Model file for the job. Use its own axes, mm. A direction names the side the tool comes from. Give positions to 0.01 mm unless a question says otherwise; leave off trailing zeros. Loops run counter-clockwise (first coordinate to the right, second up) from the corner with the lowest first, then second, coordinate; pieces in that order, holes last. Notation, with made-up numbers: M -39,-22.75 L -33,-22.75 A19 cw -33,6.25 Z; hole C 9,67 d1. An arc over 180 degrees is marked long. Use CSV: the item, a comma, the result in double quotes. Start each with the question number.
(1) Slice it at C-C on z = 15.75. List the corners of the cut face in (x, y).
(2) Wall check: line 1 along Y through (x, z) = (0, 26.1); line 2 along X through (y, z) = (-9.25, 25.65); line 3 along Y through (x, z) = (-30, 0.9). Give the ranges that are in metal, low to high. Write a range as from..to.
(3) Slice it at D-D on y = 0. State how many separate pieces and enclosed holes the cut face has, and give its area (3 significant figures).
(4) Two-plate mould, pull along Z, no slides. Class faces 4 (the face through (-15, -15, 0)), 5 (the face through (16, -16, 20)), 6 (the face through (0, -5, 28)), 7 (the face through (6.25, 0.07, 26.52)): pulls with the +Z half, pulls with the -Z half, needs draft (parallel to the pull), parting line crosses it, or undercut.
(5) Tool access for faces 1 (the face through (10.042, -20.649, 22.465)), 2 (the face through (-4, 4, 25)), 3 (the face through (-7.5, -22, 11)): list every direction of +Z, -Z, +X, -X, +Y, -Y with a clear straight run to the whole face (end or side of a thin tool).
(6) Slice it at A-A on x = 30. List the corners of the cut face in (y, z), and give its area (3 significant figures).
(7) Flat gauge pins, fed straight in: P1, Ø4, axis at y = -5.5, z = 3, coming from the -X side; P2, Ø4, axis at x = 4.5, z = 4, coming from the -Y side; P3, Ø3.5, axis at x = 0, y = -9.25, coming from the -Z side; P4, Ø7, axis at x = 0, y = 0, coming from the +Z side. Where does each tip first touch, or does it go through?
```python
from build123d import *

# Parameters (mm, degrees)
SKETCH_1_R               = 25
SKETCH_1_R_2             = 21
EXTRUDE_1_DEPTH          = 25
SKETCH_2_R               = 25
EXTRUDE_2_DEPTH          = 3
SKETCH_3_R               = 4.25
SKETCH_3_R_2             = 1.5
CUT_EXTRUDE_1_DEPTH      = 3
CUT_EXTRUDE_2_DEPTH      = 3
SKETCH_6_W               = 15
SKETCH_6_H               = 5
CUT_EXTRUDE_3_DEPTH      = 63
SKETCH_8_W               = 5
SKETCH_8_H               = 15
CUT_EXTRUDE_4_DEPTH      = 63
SKETCH_9_W               = 5
SKETCH_9_H               = 15
CUT_EXTRUDE_5_DEPTH      = 63
PATTERN_CIRCULAR_2_COUNT = 4
SKETCH_10_R              = 35
SKETCH_10_R_2            = 21
EXTRUDE_3_DEPTH          = 3
SKETCH_11_R              = 2
CUT_EXTRUDE_6_DEPTH      = 3
FILLET_1_R               = 2


with BuildPart() as part:
    # 草图1 → 凸台-拉伸1 (new body)
    with BuildSketch(Plane.XY):
        Circle(SKETCH_1_R)
        Circle(SKETCH_1_R_2, mode=Mode.SUBTRACT)
    extrude(amount=EXTRUDE_1_DEPTH)

    # 草图2 → 凸台-拉伸2 (add)
    with BuildSketch(Plane.XY.offset(25)):
        Circle(SKETCH_2_R)
    extrude(amount=EXTRUDE_2_DEPTH)

    # 草图3 → 切除-拉伸1 (cut)
    with BuildSketch(Plane.XY.offset(28)):
        Circle(SKETCH_3_R)
        with Locations((0, 9.25)):
            Circle(SKETCH_3_R_2)
        with Locations((7.75, 0)):
            Circle(SKETCH_3_R_2)
        with Locations(Location((0, -9.25, 0), (0, 0, 180))):
            Circle(SKETCH_3_R_2)
        with Locations(Location((-7.75, 0, 0), (0, 0, 180))):
            Circle(SKETCH_3_R_2)
    extrude(amount=-CUT_EXTRUDE_1_DEPTH, mode=Mode.SUBTRACT)

    # 草图4 → 切除-拉伸2 (cut)
    with BuildSketch(Plane.XY.offset(28)):
        with BuildLine():
            ThreePointArc((-17.320508076, 10), (-20, 0), (-17.320508076, -10))
            ThreePointArc((-17.320508076, -10), (-13.905444566, -10.915063509), (-12.990381057, -7.5))
            ThreePointArc((-12.990381057, -7.5), (-15, 0), (-12.990381057, 7.5))
            ThreePointArc((-12.990381057, 7.5), (-13.905444566, 10.915063509), (-17.320508076, 10))
        make_face()
        with BuildLine():
            ThreePointArc((17.320508076, 10), (20, 0), (17.320508076, -10))
            ThreePointArc((17.320508076, -10), (13.905444566, -10.915063509), (12.990381057, -7.5))
            ThreePointArc((12.990381057, -7.5), (15, 0), (12.990381057, 7.5))
            ThreePointArc((12.990381057, 7.5), (13.905444566, 10.915063509), (17.320508076, 10))
        make_face()
    extrude(amount=-CUT_EXTRUDE_2_DEPTH, mode=Mode.SUBTRACT)

    # 草图6 → 切除-拉伸3 (cut)
    with BuildSketch(Plane(origin=(17.67766953, 17.67766953, 28), x_dir=(0.7071067811865488, -0.7071067811865464, 0), z_dir=(0.7071067811865464, 0.7071067811865488, 0))):
        with Locations((0, 5.5)):
            Rectangle(SKETCH_6_W, SKETCH_6_H)
    extrude(amount=-CUT_EXTRUDE_3_DEPTH, mode=Mode.SUBTRACT)

    # 草图8 → 切除-拉伸4 (cut)
    with BuildSketch(Plane(origin=(-17.67766953, 17.67766953, 28), x_dir=(0, 0, 1), z_dir=(-0.7071067811865517, 0.7071067811865435, 0))):
        with Locations((-5.5, 0)):
            Rectangle(SKETCH_8_W, SKETCH_8_H)
    extrude(amount=-CUT_EXTRUDE_4_DEPTH, mode=Mode.SUBTRACT)

    # 草图9 → 切除-拉伸5 (cut)
    with BuildSketch(Plane(origin=(0, 0, 0), x_dir=(0, 0, -1), z_dir=(1, 0, 0))):
        with Locations((-10.5, 0)):
            Rectangle(SKETCH_9_W, SKETCH_9_H)
    cut_extrude_5 = extrude(amount=-CUT_EXTRUDE_5_DEPTH, mode=Mode.SUBTRACT)

    # 阵列(圆周)2: 切除-拉伸5 ×4 about axis
    pattern_circular_2_axis = Axis((0, 0, 0), (0, 0, 1))
    for i in range(1, PATTERN_CIRCULAR_2_COUNT):
        add(cut_extrude_5.rotate(pattern_circular_2_axis, i * 360 / PATTERN_CIRCULAR_2_COUNT), mode=Mode.SUBTRACT)

    # 草图10 → 凸台-拉伸3 (add)
    with BuildSketch(Plane(origin=(0, 0, 0), x_dir=(-1, 0, 0), z_dir=(0, 0, -1))):
        Circle(SKETCH_10_R)
        with Locations(Location((0, 0, 0), (0, 0, 24.075167572))):
            Circle(SKETCH_10_R_2, mode=Mode.SUBTRACT)
    extrude(amount=-EXTRUDE_3_DEPTH)

    # 草图11 → 切除-拉伸6 (cut)
    with BuildSketch(Plane(origin=(0, 0, 0), x_dir=(-1, 0, 0), z_dir=(0, 0, -1))):
        with Locations((0, 30)):
            Circle(SKETCH_11_R)
        with Locations((30, 0)):
            Circle(SKETCH_11_R)
        with Locations((0, -30)):
            Circle(SKETCH_11_R)
        with Locations((-30, 0)):
            Circle(SKETCH_11_R)
    extrude(amount=-CUT_EXTRUDE_6_DEPTH, mode=Mode.SUBTRACT)

    # 圆角1
    fillet_1_edges = [part.edges().sort_by_distance(p)[0] for p in [
        (-25, 0, 3),
    ]]
    fillet(fillet_1_edges, radius=FILLET_1_R)


solid = part.part
```
Reply:
1,outline,"C 0,0 d50; hole C 0,0 d42"
2,line 1,"y = -25..-10.75, -7.75..-4.25, 4.25..7.75, 10.75..25"
2,line 2,"x = -23.23..-17.73, -12.71..-1.5, 1.5..12.71, 17.73..23.23"
2,line 3,"y = -18.03..-2, 2..18.03"
3,separate pieces,"10"
3,enclosed holes,"0"
3,area,"274 mm^2"
4,face 4,"pulls with the -Z half"
4,face 5,"undercut"
4,face 6,"pulls with the +Z half"
4,face 7,"needs draft"
5,face 1,"+X"
5,face 2,"none"
5,face 3,"+Y, -Y"
6,outline,"M -18.03,0 L -2,0 L -2,3 L -18.03,3 Z; M 2,0 L 18.03,0 L 18.03,3 L 2,3 Z"
6,area,"96.2 mm^2"
7,P1,"stops at x = -34.82"
7,P2,"stops at y = -34.89"
7,P3,"stops at z = 25"
7,P4,"passes through"
